Read the model definition and answer for the solid it produces. Units are mm, in the model's axes. Face numbers are marked on the shaded views. A direction names the side the tool comes from. Give positions to 0.01 mm unless a question says otherwise; leave off trailing zeros. Order: outer loops, then holes, each group sorted by start corner. A loop starts at its lowest first (then second) coordinate and runs counter-clockwise, first axis right, second up. Notation, with made-up numbers: (-25, 41.5) - (-5, 41.5) arc R26 ccw to (-5, 75.5) - close; hole circle Ø11 at (-5, 70). An arc over 180 degrees is marked (long way). Use a Markdown table: item, result. Add a question column.
1. For a pull along Y with two mould halves and no side action, classify the marked faces 1, 2 and 3 as released by +Y, released by -Y, zero draft, split by the parting line, or undercut.
2. Consider L1, parallel to Y at x = -7, z = 17.5; L2, parallel to Z at x = 0, y = 13.05; L3, parallel to Z at x = 0, y = 13.4. Determine where each line is inside the solid, lowest interval first.
3. A cutting plane is placed at A-A on y = -5. Determine the outline of the cut face in (x, z).
4. A cutting plane is placed at B-B on z = 20. Determine the outline of the cut face in (x, y).
5. Flat-ended cylindrical pins translate along their axes: P1, Ø8, axis at x = -8, y = 0, coming from the +Z side; P2, Ø10, axis at y = -1, z = 12.5, coming from the -X side; P3, Ø10, axis at x = 2, z = 16, coming from the -Y side. Find the tip coordinate at first contact, or state that the pin passes through.
6. Which of the six approach directions +Z, -Z, +X, -X, +Y, -Y give full straight-line access (tool end or side, diameter ignored) to the marked faces 4 and 5?
7. A cutting plane is placed at C-C on x = 0. State how many separate pieces and enclosed holes the cut face has, and give its area (3 significant figures).
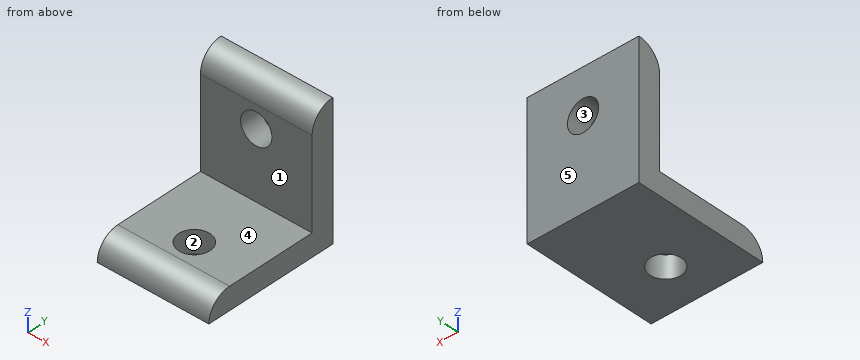
```python
from build123d import *

# Parameters (mm, degrees)
F0_W     = 25
F0_H     = 25
F0_R     = 3.5
F1_DEPTH = 5
F0_H_2   = 5
F2_DEPTH = 30
F3_R     = 3.5
F4_DEPTH = 5
F5_R     = 4.99999
F6_R     = 4.99999


# Not quite as in the source:
# - a fillet or chamfer is up to 0.001 mm smaller than in the source, because OpenCascade refuses the exact size


with BuildPart() as f1:
    # F0 (on Top) → F1 (new body)
    with BuildSketch(Plane.XY):
        with Locations((0, -2.5)):
            Rectangle(F0_W, F0_H)
        with Locations((0, -5)):
            Circle(F0_R, mode=Mode.SUBTRACT)
    extrude(amount=F1_DEPTH)

    # F0 (on Top) → F2 (join)
    with BuildSketch(Plane.XY):
        with Locations((0, 12.5)):
            Rectangle(F0_W, F0_H_2)
    extrude(amount=F2_DEPTH)

    # F3 (on face) → F4 (cut)
    with BuildSketch(Plane(origin=(0, 15, 0), x_dir=(-1, 0, 0), z_dir=(0, 1, 0))):
        with Locations((0, 20)):
            Circle(F3_R)
    extrude(amount=-F4_DEPTH, mode=Mode.SUBTRACT)

    # F5 (radius 5 in the source; OpenCascade refuses exactly that, so slightly less here)
    f5_edges = [f1.edges().sort_by_distance(p)[0] for p in [
        (0, 10, 30),
    ]]
    fillet(f5_edges, radius=F5_R)

    # F6 (radius 5 in the source; OpenCascade refuses exactly that, so slightly less here)
    f6_edges = [f1.edges().sort_by_distance(p)[0] for p in [
        (0, -15, 5),
    ]]
    fillet(f6_edges, radius=F6_R)


solid = f1.part
```
Output values:
| question | item | result |
|---|---|---|
| 1 | face 1 | released by -Y |
| 1 | face 2 | undercut |
| 1 | face 3 | zero draft |
| 2 | L1 | 10 to 15 |
| 2 | L2 | 0 to 16.5, 23.5 to 29.6 |
| 2 | L3 | 0 to 16.5, 23.5 to 29.74 |
| 3 | outline | (-12.5, 0) - (-3.5, 0) - (-3.5, 5) - (-12.5, 5) - close; (3.5, 0) - (12.5, 0) - (12.5, 5) - (3.5, 5) - close |
| 4 | outline | (-12.5, 10) - (-3.5, 10) - (-3.5, 15) - (-12.5, 15) - close; (3.5, 10) - (12.5, 10) - (12.5, 15) - (3.5, 15) - close |
| 5 | P1 | z = 5 |
| 5 | P2 | through |
| 5 | P3 | y = 10 |
| 6 | face 4 | +Z, +X, -X, -Y |
| 6 | face 5 | +Z, -Z, +X, -X, +Y |
| 7 | separate pieces | 3 |
| 7 | enclosed holes | 0 |
| 7 | area | 194 mm² |
